```python
from build123d import *

# Parameters (mm, degrees)
SKETCH1_W            = 184
SKETCH1_H            = 165
BOSS_EXTRUDE1_DEPTH  = 4
M5_CLEARANCE_HOLE1_D = 5.5
SKETCH4_W            = 80
SKETCH4_H            = 30
CUT_EXTRUDE1_DEPTH   = 10
SKETCH5_W            = 52
SKETCH5_H            = 60
SKETCH5_H_2          = 30
BOSS_EXTRUDE2_DEPTH  = 4
M5_CLEARANCE_HOLE2_D = 5.5


with BuildPart() as part:
    # Sketch1 → Boss-Extrude1 (new body)
    with BuildSketch(Plane.XY):
        with Locations((70, 60)):
            Rectangle(SKETCH1_W, SKETCH1_H)
    extrude(amount=BOSS_EXTRUDE1_DEPTH)

    # M5 Clearance Hole1 (through all)
    with Locations(Plane(origin=(0, 0, 0), x_dir=(-1, 0, 0), z_dir=(0, 0, -1))):
        with Locations((-16, -15), (-16, 15), (16, 15), (16, -15), (16, 105), (-16, 105), (-16, 135), (16, 135), (-124, 135), (-124, 105), (-156, 105), (-156, 135), (-156, 15), (-124, 15), (-124, -15), (-156, -15)):
            Hole(M5_CLEARANCE_HOLE1_D / 2)

    # Sketch4 → Cut-Extrude1 (cut)
    with BuildSketch(Plane.XY.offset(4)):
        with Locations((70, -7.5)):
            Rectangle(SKETCH4_W, SKETCH4_H)
    extrude(amount=-CUT_EXTRUDE1_DEPTH, mode=Mode.SUBTRACT)

    # Sketch5 → Boss-Extrude2 (add)
    with BuildSketch(Plane.XY.offset(4)):
        with Locations((136, -52.5)):
            Rectangle(SKETCH5_W, SKETCH5_H)
        with Locations((136, 157.5)):
            Rectangle(SKETCH5_W, SKETCH5_H_2)
    extrude(amount=-BOSS_EXTRUDE2_DEPTH)

    # M5 Clearance Hole2 (through all)
    with Locations(Plane.XY.offset(4)):
        with Locations((149.5, -67.5), (124.5, -67.5), (124.5, 157.5), (149.5, 157.5)):
            Hole(M5_CLEARANCE_HOLE2_D / 2)


solid = part.part
```
Check sheet for the modelled part. Datum: model origin and axes. Units: mm. Give positions to 0.01 mm unless a question says otherwise; leave off trailing zeros. Write each loop counter-clockwise with the first axis right and the second up, starting at its lowest first coordinate (ties: lowest second). Pieces come first, ordered by that corner, then holes.
Item 1: Gauge pin test, flat ends, axial feed: pin 1 (9 mm diameter, centred on x = 124, y = 105, fed in from +Z); pin 2 (2 mm diameter, centred on x = 34, z = 2.5, fed in from +Y); pin 3 (1.2 mm diameter, centred on x = 84.5, z = 1, fed in from -Y); pin 4 (1.5 mm diameter, centred on y = -34.5, z = 1.5, fed in from -X). Record the tip position at first contact, or that the pin passes through.
Item 2: Cross-section at A-A (x = 149.5). Enter the section's corners in (y, z), and give its area (3 significant figures).
Item 3: Cross-section at C-C (z = 0.8). Count the separate pieces of the cut face and the enclosed holes in it, and give its area (3 significant figures).
Item 4: Scan lines: L1, parallel to Y at x = 156, z = 3.05; L2, parallel to Y at x = -16, z = 1; L3, parallel to Y at x = 149.5, z = 1.25. Record each from-to range of solid material in increasing order.
Item 5: Cross-section at B-B (y = 157.5). Enter the section's corners in (x, z), and give its area (3 significant figures).
Item 6: Cross-section at D-D (x = -16). Enter the section's corners in (y, z), and give its area (3 significant figures).
Item 7: Draft check along Y on faces 1 (the face through (158.54, 103.95, 2.03)), 2 (the face through (69, 75, 0)). Enter one of: released by +Y, released by -Y, zero draft, split by the parting line, or undercut.
Report:
1. pin 1: stops at z = 4
1. pin 2: stops at y = 142.5
1. pin 3: stops at y = 7.5
1. pin 4: stops at x = 110
2. outline: (-82.5, 0) - (-70.25, 0) - (-70.25, 4) - (-82.5, 4) - close; (-64.75, 0) - (154.75, 0) - (154.75, 4) - (-64.75, 4) - close; (160.25, 0) - (172.5, 0) - (172.5, 4) - (160.25, 4) - close
2. area: 976 mm2
3. separate pieces: 1
3. enclosed holes: 20
3. area: 32,200 mm2
4. L1: y = -82.5 to -17.75, -12.25 to 12.25, 17.75 to 102.25, 107.75 to 132.25, 137.75 to 172.5
4. L2: y = -22.5 to -17.75, -12.25 to 12.25, 17.75 to 102.25, 107.75 to 132.25, 137.75 to 142.5
4. L3: y = -82.5 to -70.25, -64.75 to 154.75, 160.25 to 172.5
5. outline: (110, 0) - (121.75, 0) - (121.75, 4) - (110, 4) - close; (127.25, 0) - (146.75, 0) - (146.75, 4) - (127.25, 4) - close; (152.25, 0) - (162, 0) - (162, 4) - (152.25, 4) - close
5. area: 164 mm2
6. outline: (-22.5, 0) - (-17.75, 0) - (-17.75, 4) - (-22.5, 4) - close; (-12.25, 0) - (12.25, 0) - (12.25, 4) - (-12.25, 4) - close; (17.75, 0) - (102.25, 0) - (102.25, 4) - (17.75, 4) - close; (107.75, 0) - (132.25, 0) - (132.25, 4) - (107.75, 4) - close; (137.75, 0) - (142.5, 0) - (142.5, 4) - (137.75, 4) - close
6. area: 572 mm2
7. face 1: undercut
7. face 2: zero draft
